Can you work these out from the model? Positions are in its coordinate system, mm. Face numbers are marked on the shaded views. Coordinates: 2 decimals unless noted, no trailing zeros. Write each loop counter-clockwise with the first axis right and the second up, starting at its lowest first coordinate (ties: lowest second). Pieces come first, ordered by that corner, then holes. Notation, with made-up numbers: (-10, -21) - (22, -21) arc R17 ccw to (22, -5) - close; hole circle Ø9 at (-21.5, 49). An arc over 180 degrees is marked (long way). Use one line per item in the form item = value. Start each with the question number.
(1) Thinking about a two-plate mould opening in Z: for the marked faces 1, 2 and 3, which applies, pulls with the +Z half, pulls with the -Z half, needs draft (parallel to the pull), parting line crosses it, or undercut?
(2) If we section it at D-D on z = 0.7: Please give me the cut outline in (x, y), then the cut area to 3 significant figures.
(3) If we section it at B-B on x = 0: Please give me the cut outline in (y, z), then the cut area to 3 significant figures.
(4) If I drill on probe 1 along Z at (x, y) = (8.75, 1.5); probe 2 along Y at (x, z) = (0, 0.4); probe 3 along Z at (x, y) = (2.75, 8), over which ranges is the centre line in solid material (lowest first)? Write a range as from..to.
(5) For pin 1 Ø1.5 at (x, z) = (5, -0.5) entering from -Y, with a flat end and sliding along its axis, tell me the tip position at first contact or that it passes through.
(6) If we section it at C-C on z = 0.05: Please give me the cut outline in (x, y).
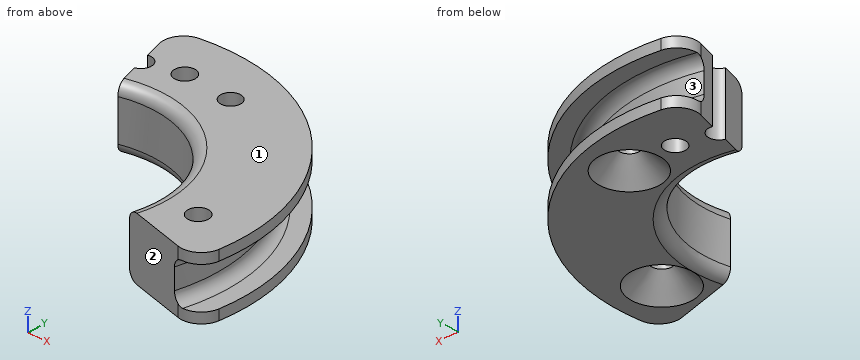
```python
from build123d import *

# Parameters (mm, degrees)
SKETCH1_R               = 8.5
SKETCH1_R_2             = 0.5
SKETCH1_R_3             = 5
BOSS_EXTRUDE1_DEPTH     = 1.5
SKETCH7_W               = 0.8
SKETCH7_H               = 0.5
CUT_EXTRUDE1_DEPTH      = 14.237446884
CUT_EXTRUDE1_DEPTH_BACK = 14.237446884
CUT_EXTRUDE2_DEPTH      = 14.489996294
CUT_EXTRUDE2_DEPTH_BACK = 14.489996294
SKETCH5_R               = 0.5
SKETCH5_R_2             = 0.48729794
FILLET1_R               = 0.5
FILLET2_R               = 1
CHAMFER1_SIZE           = 1


with BuildPart() as part:
    # Sketch1 → Boss-Extrude1 (new, symmetric)
    with BuildSketch(Plane.XY):
        Circle(SKETCH1_R)
        with Locations((7, 0)):
            Circle(SKETCH1_R_2, mode=Mode.SUBTRACT)
        Circle(SKETCH1_R_3, mode=Mode.SUBTRACT)
        with Locations((0, -7)):
            Circle(SKETCH1_R_2, mode=Mode.SUBTRACT)
        with Locations((-7, 0)):
            Circle(SKETCH1_R_2, mode=Mode.SUBTRACT)
        with Locations((0, 7)):
            Circle(SKETCH1_R_2, mode=Mode.SUBTRACT)
    extrude(amount=BOSS_EXTRUDE1_DEPTH, both=True)

    # Sketch2 → Cut-Revolve1 (revolve, cut)
    with BuildSketch(Plane(origin=(0, 0, 0), x_dir=(1, 0, 0), z_dir=(0, 1, 0)), mode=Mode.PRIVATE) as cut_revolve1_sk:
        with BuildLine():
            Line((-8, 0.5), (-8, -0.5))
            ThreePointArc((-8, -0.5), (-8.146446609, -0.853553391), (-8.5, -1))
            Line((-8.5, -1), (-8.5, 1))
            ThreePointArc((-8.5, 1), (-8.146446609, 0.853553391), (-8, 0.5))
        make_face()
    revolve(cut_revolve1_sk.sketch.rotate(Axis((0, 0, 0), (0, 0, -1)), 180), axis=Axis((0, 0, 0), (0, 0, -1)), mode=Mode.SUBTRACT)

    # Sketch7 → Revolve1 (revolve)
    with BuildSketch(Plane(origin=(0, 0, 0), x_dir=(1, 0, 0), z_dir=(0, 1, 0))):
        with Locations((8.9, 1.25)):
            Rectangle(SKETCH7_W, SKETCH7_H)
        with Locations((8.9, -1.25)):
            Rectangle(SKETCH7_W, SKETCH7_H)
    revolve(axis=Axis((0, 0, 0), (0, 0, -1)))

    # Sketch4 → Cut-Extrude1 (cut, two sides: drawn at the far end of the back side and taken through both)
    with BuildSketch(Plane.XY.offset(-CUT_EXTRUDE1_DEPTH_BACK)):
        Polygon((-2.654263152, 9.905844942), (0, 0), (10.350145374, -2.773313095), (10.350145374, -11.033622271), (-11.334173843, -11.033622271), (-11.334173843, 9.905844942), align=None)
    extrude(amount=CUT_EXTRUDE1_DEPTH + CUT_EXTRUDE1_DEPTH_BACK, mode=Mode.SUBTRACT)

    # Sketch5 → Cut-Extrude2 (cut, two sides: drawn at the far end of the back side and taken through both)
    with BuildSketch(Plane.XY.offset(1.5).offset(-CUT_EXTRUDE2_DEPTH_BACK)):
        with Locations((-1.768253171, 6.599210675)):
            Circle(SKETCH5_R)
        with Locations((2.418011057, 6.794599377)):
            Circle(SKETCH5_R_2)
    extrude(amount=CUT_EXTRUDE2_DEPTH + CUT_EXTRUDE2_DEPTH_BACK, mode=Mode.SUBTRACT)

    # Fillet1
    fillet1_edges = [part.edges().sort_by_distance(p)[0] for p in [
        (3.535533906, 3.535533906, 1.5),
        (3.535533906, 3.535533906, -1.5),
    ]]
    fillet(fillet1_edges, radius=FILLET1_R)

    # Fillet2
    fillet2_edges = [part.edges().sort_by_distance(p)[0] for p in [
        (8.983110184, -2.407017119, -1.25),
        (8.983110184, -2.407017119, 1.25),
        (-2.407017119, 8.983110184, -1.25),
        (-2.407017119, 8.983110184, 1.25),
    ]]
    fillet(fillet2_edges, radius=FILLET2_R)

    # Chamfer1
    chamfer1_edges = [part.edges().sort_by_distance(p)[0] for p in [
        (6.5, 0, -1.5),
        (1.930713118, 6.794599377, -1.5),
    ]]
    chamfer(chamfer1_edges, length=CHAMFER1_SIZE - 0.0001)  # a hair under: the kernel refuses the full size


solid = part.part
```
Reported:
q1.face_1 = pulls with the +Z half
q1.face_2 = needs draft
q1.face_3 = undercut
q2.outline = (-2.08, 7.77) - (-1.9, 7.08) arc R0.5 cw to (-1.64, 6.12) - (-1.29, 4.83) arc R5 cw to (4.83, -1.29) - (7.77, -2.08) arc R8.04 ccw to start; hole circle Ø1 at (0, 7); hole circle Ø0.97 at (2.42, 6.79); hole circle Ø1 at (7, 0)
q2.area = 38.8 mm2
q3.outline = (5, -1) arc R0.5 ccw to (5.5, -1.5) - (6.5, -1.5) - (6.5, 1.5) - (5.5, 1.5) arc R0.5 ccw to (5, 1) - close; (7.5, -1.5) - (9.3, -1.5) - (9.3, -1) - (8.5, -1) arc R0.5 cw to (8, -0.5) - (8, 0.5) arc R0.5 cw to (8.5, 1) - (9.3, 1) - (9.3, 1.5) - (7.5, 1.5) - close
q3.area = 7.30 mm2
q4.probe_1 = -1.5..-1, 1..1.5
q4.probe_2 = 5..6.5, 7.5..8
q4.probe_3 = -1.26..-1, 1..1.5
q5.pin_1 = -1.54
q6.outline = (-2.07, 7.73) - (-1.9, 7.08) arc R0.5 cw to (-1.64, 6.12) - (-1.29, 4.83) arc R5 cw to (4.83, -1.29) - (7.73, -2.07) arc R8 ccw to start; hole circle Ø1 at (0, 7); hole circle Ø0.97 at (2.42, 6.79); hole circle Ø1 at (7, 0)
